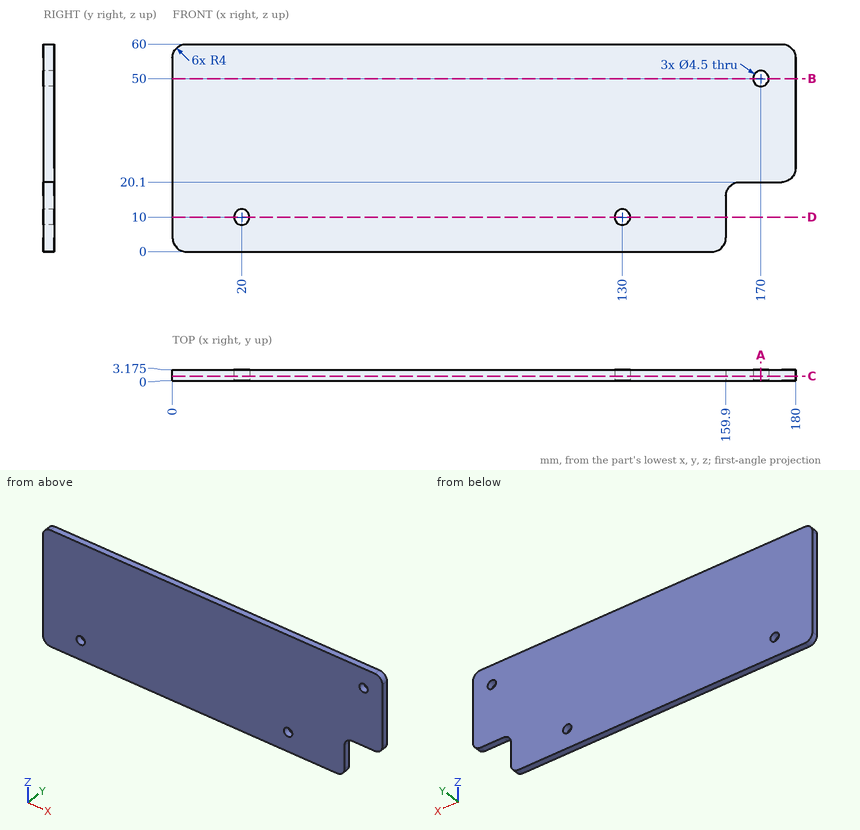
Print and shaded views of the part. All mm, measured from the part's lowest x, y and z. Give positions to 0.01 mm unless a question says otherwise; leave off trailing zeros. Loops run counter-clockwise (first coordinate to the right, second up) from the corner with the lowest first, then second, coordinate; pieces in that order, holes last. Notation, with made-up numbers: (-0.75, 88) - (21.25, 88) arc R27 ccw to (21.25, 124) - close; hole circle Ø9 at (50.25, 18.5). An arc over 180 degrees is marked (long way). One line per item, written item: value. Start each with the question number.
1. Slice it at C-C (y = 1.3). List the corners of the cut face in (x, z).
2. Slice it at D-D (z = 10). List the corners of the cut face in (x, y) (3 decimals), plus the area to 3 significant figures.
3. Slice it at B-B (z = 50). List the corners of the cut face in (x, y) (3 decimals).
4. Slice it at A-A (x = 170). List the corners of the cut face in (y, z) (3 decimals), plus the area to 3 significant figures.
5. Probe L1, parallel to X at y = 1.85, z = 10; L2, parallel to X at y = 1.7, z = 50; L3, parallel to Z at x = 20, y = 1.2. List the from-to ranges inside material, lowest first. Write a range as from..to.
6. Pin check, flat tips, straight feed: pin 1 (12 mm diameter, centred on x = 154, z = 10.5, fed in from -Y); pin 2 (1 mm diameter, centred on y = 2, z = 10.5, fed in from +X); pin 3 (1.6 mm diameter, centred on x = 172, y = 1.5, fed in from -Z). Stop position of each tip, or through.
Solution:
1. outline: (0, 4) arc R4 ccw to (4, 0) - (155.9, 0) arc R4 ccw to (159.9, 4) - (159.9, 16.1) arc R4 cw to (163.9, 20.1) - (176, 20.1) arc R4 ccw to (180, 24.1) - (180, 56) arc R4 ccw to (176, 60) - (4, 60) arc R4 ccw to (0, 56) - close; hole circle Ø4.5 at (20, 10); hole circle Ø4.5 at (130, 10); hole circle Ø4.5 at (170, 50)
2. outline: (0, 0) - (17.75, 0) - (17.75, 3.175) - (0, 3.175) - close; (22.25, 0) - (127.75, 0) - (127.75, 3.175) - (22.25, 3.175) - close; (132.25, 0) - (159.9, 0) - (159.9, 3.175) - (132.25, 3.175) - close
2. area: 479 mm^2
3. outline: (0, 0) - (167.75, 0) - (167.75, 3.175) - (0, 3.175) - close; (172.25, 0) - (180, 0) - (180, 3.175) - (172.25, 3.175) - close
4. outline: (0, 20.1) - (3.175, 20.1) - (3.175, 47.75) - (0, 47.75) - close; (0, 52.25) - (3.175, 52.25) - (3.175, 60) - (0, 60) - close
4. area: 112 mm^2
5. L1: x = 0..17.75, 22.25..127.75, 132.25..159.9
5. L2: x = 0..167.75, 172.25..180
5. L3: z = 0..7.75, 12.25..60
6. pin 1: stops at y = 0
6. pin 2: stops at x = 159.9
6. pin 3: stops at z = 20.1
